```python
from build123d import *

# Parameters (mm, degrees)
SALIENTE_EXTRUIR1_DEPTH = 6.5
CROQUIS2_R              = 9.95
CORTAR_EXTRUIR1_DEPTH   = 4.5
CROQUIS3_R              = 3.5
CROQUIS3_R_2            = 1.025
CORTAR_EXTRUIR2_DEPTH   = 3.5
SALIENTE_EXTRUIR2_DEPTH = 16
SALIENTE_EXTRUIR3_DEPTH = 8
CORTAR_EXTRUIR3_DEPTH   = 8
CROQUIS8_R              = 1.5
CORTAR_EXTRUIR4_DEPTH   = 44.411432826
CROQUIS9_W              = 3.5
CROQUIS9_H              = 30.5
CORTAR_EXTRUIR6_DEPTH   = 44.411432826
REDONDEO4_R             = 3
REDONDEO5_R             = 1


with BuildPart() as part:
    # Croquis1 → Saliente-Extruir1 (new body)
    with BuildSketch(Plane.XY):
        with BuildLine():
            Line((-13.869120376, 1.5), (-24, 1.5))
            Line((-24, 1.5), (-24, 5.5))
            Line((-24, 5.5), (-12.8200039, 5.5))
            ThreePointArc((-12.8200039, 5.5), (0, 13.95), (12.8200039, 5.5))
            Line((12.8200039, 5.5), (24, 5.5))
            Line((24, 5.5), (24, 1.5))
            Line((24, 1.5), (13.869120376, 1.5))
            ThreePointArc((13.869120376, 1.5), (13.95, 0), (13.869120376, -1.5))
            Line((13.869120376, -1.5), (24, -1.5))
            Line((24, -1.5), (24, -5.5))
            Line((24, -5.5), (12.8200039, -5.5))
            ThreePointArc((12.8200039, -5.5), (0, -13.95), (-12.8200039, -5.5))
            Line((-12.8200039, -5.5), (-24, -5.5))
            Line((-24, -5.5), (-24, -1.5))
            Line((-24, -1.5), (-13.869120376, -1.5))
            ThreePointArc((-13.869120376, -1.5), (-13.95, 0), (-13.869120376, 1.5))
        make_face()
    extrude(amount=SALIENTE_EXTRUIR1_DEPTH)

    # Croquis2 → Cortar-Extruir1 (cut)
    with BuildSketch(Plane.XY.offset(6.5)):
        Circle(CROQUIS2_R)
    extrude(amount=-CORTAR_EXTRUIR1_DEPTH, mode=Mode.SUBTRACT)

    # Croquis3 → Cortar-Extruir2 (cut)
    with BuildSketch(Plane.XY.offset(2)):
        Circle(CROQUIS3_R)
        with Locations((-7.5, 0)):
            Circle(CROQUIS3_R_2)
        with Locations((7.5, 0)):
            Circle(CROQUIS3_R_2)
    extrude(amount=-CORTAR_EXTRUIR2_DEPTH, mode=Mode.SUBTRACT)

    # Croquis4 → Saliente-Extruir2 (add)
    with BuildSketch(Plane.XY.offset(6.5)):
        with BuildLine():
            Line((-12.8200039, 5.5), (-24, 5.5))
            Line((-24, 5.5), (-24, 1.5))
            Line((-24, 1.5), (-13.869120376, 1.5))
            ThreePointArc((-13.869120376, 1.5), (-13.49360362, 3.539090469), (-12.8200039, 5.5))
        make_face()
        with BuildLine():
            Line((-13.869120376, -1.5), (-24, -1.5))
            Line((-24, -1.5), (-24, -5.5))
            Line((-24, -5.5), (-12.8200039, -5.5))
            ThreePointArc((-12.8200039, -5.5), (-13.49360362, -3.539090469), (-13.869120376, -1.5))
        make_face()
        with BuildLine():
            Line((24, -5.5), (12.8200039, -5.5))
            ThreePointArc((12.8200039, -5.5), (13.49360362, -3.539090469), (13.869120376, -1.5))
            Line((13.869120376, -1.5), (24, -1.5))
            Line((24, -1.5), (24, -5.5))
        make_face()
        with BuildLine():
            Line((24, 1.5), (13.869120376, 1.5))
            ThreePointArc((13.869120376, 1.5), (13.49360362, 3.539090469), (12.8200039, 5.5))
            Line((12.8200039, 5.5), (24, 5.5))
            Line((24, 5.5), (24, 1.5))
        make_face()
    extrude(amount=SALIENTE_EXTRUIR2_DEPTH)

    # Croquis6 → Saliente-Extruir3 (add)
    with BuildSketch(Plane.XY.offset(22.5)):
        with BuildLine():
            Line((-12.8200039, 5.5), (-24, 5.5))
            Line((-24, 5.5), (-24, 1.5))
            Line((-24, 1.5), (-13.869120376, 1.5))
            ThreePointArc((-13.869120376, 1.5), (-13.95, 0), (-13.869120376, -1.5))
            Line((-13.869120376, -1.5), (-24, -1.5))
            Line((-24, -1.5), (-24, -5.5))
            Line((-24, -5.5), (-12.8200039, -5.5))
            ThreePointArc((-12.8200039, -5.5), (0, -13.95), (12.8200039, -5.5))
            Line((12.8200039, -5.5), (24, -5.5))
            Line((24, -5.5), (24, -1.5))
            Line((24, -1.5), (13.869120376, -1.5))
            ThreePointArc((13.869120376, -1.5), (13.95, 0), (13.869120376, 1.5))
            Line((13.869120376, 1.5), (24, 1.5))
            Line((24, 1.5), (24, 5.5))
            Line((24, 5.5), (12.8200039, 5.5))
            ThreePointArc((12.8200039, 5.5), (0, 13.95), (-12.8200039, 5.5))
        make_face()
    extrude(amount=SALIENTE_EXTRUIR3_DEPTH)

    # Croquis7 → Cortar-Extruir3 (cut)
    with BuildSketch(Plane.XY.offset(30.5)):
        with BuildLine():
            Line((-6.425, 7.922081482), (6.425, 7.922081482))
            ThreePointArc((6.425, 7.922081482), (10.2, 0), (6.425, -7.922081482))
            Line((6.425, -7.922081482), (-6.425, -7.922081482))
            ThreePointArc((-6.425, -7.922081482), (-10.2, 0), (-6.425, 7.922081482))
        make_face()
    extrude(amount=-CORTAR_EXTRUIR3_DEPTH, mode=Mode.SUBTRACT)

    # Croquis8 → Cortar-Extruir4 (cut, through all)
    with BuildSketch(Plane(origin=(0, 5.5, 0), x_dir=(1, 0, 0), z_dir=(0, 1, 0))):
        with Locations(Location((16.8700039, -26.5, 0), (0, 0, 180))):
            Circle(CROQUIS8_R)
        with Locations(Location((16.8700039, -4, 0), (0, 0, 180))):
            Circle(CROQUIS8_R)
        with Locations(Location((-16.8700039, -4, 0), (0, 0, 180))):
            Circle(CROQUIS8_R)
        with Locations(Location((-16.8700039, -26.5, 0), (0, 0, 180))):
            Circle(CROQUIS8_R)
    extrude(amount=-CORTAR_EXTRUIR4_DEPTH, mode=Mode.SUBTRACT)

    # Croquis9 → Cortar-Extruir6 (cut, through all)
    with BuildSketch(Plane(origin=(0, 5.5, 0), x_dir=(1, 0, 0), z_dir=(0, 1, 0))):
        with Locations((22.25, -15.25)):
            Rectangle(CROQUIS9_W, CROQUIS9_H)
        with Locations((-22.25, -15.25)):
            Rectangle(CROQUIS9_W, CROQUIS9_H)
    extrude(amount=-CORTAR_EXTRUIR6_DEPTH, mode=Mode.SUBTRACT)

    # Redondeo4
    redondeo4_edges = [part.edges().sort_by_distance(p)[0] for p in [
        (20.5, -3.5, 30.5),
        (20.5, 3.5, 30.5),
        (20.5, -3.5, 0),
        (20.5, 3.5, 0),
        (-20.5, 3.5, 30.5),
        (-20.5, -3.5, 30.5),
        (-20.5, 3.5, 0),
        (-20.5, -3.5, 0),
    ]]
    fillet(redondeo4_edges, radius=REDONDEO4_R)

    # Redondeo5
    redondeo5_edges = [part.edges().sort_by_distance(p)[0] for p in [
        (0, 13.95, 30.5),
        (-15.16000195, 5.5, 30.5),
        (0, -13.95, 30.5),
        (15.16000195, -5.5, 30.5),
        (15.16000195, -5.5, 0),
        (0, -13.95, 0),
        (-15.16000195, 5.5, 0),
        (0, 13.95, 0),
        (20.5, -5.5, 15.25),
        (-15.16000195, -5.5, 0),
        (15.16000195, 5.5, 0),
        (19.621320344, -5.5, 29.621320344),
        (19.621320344, -5.5, 0.878679656),
        (20.5, 5.5, 15.25),
        (15.16000195, 5.5, 30.5),
        (19.621320344, 5.5, 29.621320344),
        (19.621320344, 5.5, 0.878679656),
        (-15.16000195, -5.5, 30.5),
        (-20.5, -5.5, 15.25),
        (-19.621320344, -5.5, 29.621320344),
        (-19.621320344, -5.5, 0.878679656),
        (-20.5, 5.5, 15.25),
        (-19.621320344, 5.5, 29.621320344),
        (-19.621320344, 5.5, 0.878679656),
    ]]
    fillet(redondeo5_edges, radius=REDONDEO5_R)


solid = part.part
```
Part model, mm, in its own coordinate system. A direction names the side the tool comes from. Give positions to 0.01 mm unless a question says otherwise; leave off trailing zeros. Write each loop counter-clockwise with the first axis right and the second up, starting at its lowest first coordinate (ties: lowest second). Pieces come first, ordered by that corner, then holes. Notation, with made-up numbers: M 0.5,-1.75 L 45.5,-1.75 A21 cw 45.5,28.25 Z; hole C 11,11 d3. An arc over 180 degrees is marked long. Use CSV: the item, a comma, the result in double quotes.
Item 1: Slice it at B-B on z = 14.5. Write the cut outline in (x, y).
Taken from the geometry:
outline,"M -20.5,-4.5 A1 ccw -19.5,-5.5 L -12.82,-5.5 A13.95 cw -13.87,-1.5 L -20.5,-1.5 Z; M -20.5,1.5 L -13.87,1.5 A13.95 cw -12.82,5.5 L -19.5,5.5 A1 ccw -20.5,4.5 Z; M 12.82,-5.5 L 19.5,-5.5 A1 ccw 20.5,-4.5 L 20.5,-1.5 L 13.87,-1.5 A13.95 cw Z; M 12.82,5.5 A13.95 cw 13.87,1.5 L 20.5,1.5 L 20.5,4.5 A1 ccw 19.5,5.5 Z"
Item 2: Which spindle directions (+Z, -Z, +X, -X, +Y, -Y) get a long thin tool onto all of the face, cutting with end or side? Do faces 1 (the face through (19.6, 2.98, 0.86)), 2 (the face through (-10.2, -0.1, 26.6)), 3 (the face through (-14.859, 5.215, 30.199)), 4 (the face through (14.859, 5.199, 0.285)). Say none if no direction does.
Taken from the geometry:
face 1,"-Z, +X, +Y, -Y"
face 2,"+Z"
face 3,"+Z, -X, +Y"
face 4,"-Z, +X, +Y"
Item 3: Slice it at C-C on y = 0. Write the cut outline in (x, z) (3 decimals).
Taken from the geometry:
outline,"M -13.95,0 L -8.525,0 L -8.525,2 L -9.95,2 L -9.95,6.5 L -13.95,6.5 Z; M -13.95,22.5 L -10.2,22.5 L -10.2,30.5 L -13.95,30.5 Z; M -6.475,0 L -3.5,0 L -3.5,2 L -6.475,2 Z; M 3.5,0 L 6.475,0 L 6.475,2 L 3.5,2 Z; M 8.525,0 L 13.95,0 L 13.95,6.5 L 9.95,6.5 L 9.95,2 L 8.525,2 Z; M 10.2,22.5 L 13.95,22.5 L 13.95,30.5 L 10.2,30.5 Z"
Item 4: Slice it at A-A on x = 0. Write the cut outline in (y, z).
Taken from the geometry:
outline,"M -13.95,1 A1 ccw -12.95,0 L -3.5,0 L -3.5,2 L -9.95,2 L -9.95,6.5 L -13.95,6.5 Z; M -13.95,22.5 L -7.92,22.5 L -7.92,30.5 L -12.95,30.5 A1 ccw -13.95,29.5 Z; M 3.5,0 L 12.95,0 A1 ccw 13.95,1 L 13.95,6.5 L 9.95,6.5 L 9.95,2 L 3.5,2 Z; M 7.92,22.5 L 13.95,22.5 L 13.95,29.5 A1 ccw 12.95,30.5 L 7.92,30.5 Z"
Item 5: Slice it at D-D on z = 24.5. Write the cut outline in (x, y) (3 decimals), plus the area to 3 significant figures.
Taken from the geometry:
outline,"M -20.5,-4.5 A1 ccw -19.5,-5.5 L -12.82,-5.5 A13.95 ccw 12.82,-5.5 L 19.5,-5.5 A1 ccw 20.5,-4.5 L 20.5,-1.5 L 13.869,-1.5 A13.95 ccw 13.869,1.5 L 20.5,1.5 L 20.5,4.5 A1 ccw 19.5,5.5 L 12.82,5.5 A13.95 ccw -12.82,5.5 L -19.5,5.5 A1 ccw -20.5,4.5 L -20.5,1.5 L -13.869,1.5 A13.95 ccw -13.869,-1.5 L -20.5,-1.5 Z; hole M -6.425,-7.922 L 6.425,-7.922 A10.2 ccw 6.425,7.922 L -6.425,7.922 A10.2 ccw Z"
area,"436 mm²"
Item 6: Pin check, flat tips, straight feed: P1, Ø8, axis at y = 10, z = 25, coming from the -X side; P2, Ø3, axis at y = 6, z = 12.5, coming from the +X side; P3, Ø7.5, axis at x = 15, z = 17.5, coming from the -Y side; P4, Ø5.5, axis at x = 16.5, z = 21, coming from the +Y side. Stop position of each tip, or through.
Taken from the geometry:
P1,"stops at x = -12.59"
P2,"stops at x = 20.5"
P3,"stops at y = -5.5"
P4,"stops at y = 5.5"
Item 7: Pull direction Y, two halves, no side cores. Call faces 5 (the face through (14.784, 5.199, 30.215)), 6 (the face through (3.233, -1.341, 1.014)), 7 (the face through (-19.6, 2.98, 0.86)): +Y half, -Y half, draft (parallel to the pull), parting line (faces both ways), or undercut.
Taken from the geometry:
face 5,"+Y half"
face 6,"undercut"
face 7,"draft"
Item 8: Drill centre lines: probe 1 along Y at (x, z) = (-17.5, 15.5); probe 2 along Z at (x, y) = (-10.5, 7.25); probe 3 along Z at (x, y) = (-16.5, -2.75). Where is each one in solid material? Low to high.
Taken from the geometry:
probe 1,"y = -5.5 to -1.5, 1.5 to 5.5"
probe 2,"z = 0 to 6.5, 22.5 to 30.5"
probe 3,"z = 0 to 2.55, 5.45 to 25.05, 27.95 to 30.5"
